from build123d import *

# Parameters (mm, degrees)
DODANIE_WYCI_GNI_CIE1_DEPTH = 45


with BuildPart() as part:
    # Szkic1 → Dodanie-wyciągnięcie1 (new body)
    with BuildSketch(Plane(origin=(0, 0, 0), x_dir=(1, 0, 0), z_dir=(0, 1, 0))):
        with BuildLine():
            Line((0, 3.9), (2.839339828, 3.9))
            Line((2.839339828, 3.9), (5.5, 6.560660172))
            Line((5.5, 6.560660172), (5.5, 8.2))
            Line((5.5, 8.2), (3.1, 8.2))
            Line((3.1, 8.2), (3.1, 10))
            Line((3.1, 10), (8.5, 10))
            ThreePointArc((8.5, 10), (9.560660172, 9.560660172), (10, 8.5))
            Line((10, 8.5), (10, 3.1))
            Line((10, 3.1), (8.2, 3.1))
            Line((8.2, 3.1), (8.2, 5.5))
            Line((8.2, 5.5), (6.560660172, 5.5))
            Line((6.560660172, 5.5), (3.9, 2.839339828))
            Line((3.9, 2.839339828), (3.9, 0))
            Line((3.9, 0), (3.9, -2.839339828))
            Line((3.9, -2.839339828), (6.560660172, -5.5))
            Line((6.560660172, -5.5), (8.2, -5.5))
            Line((8.2, -5.5), (8.2, -3.1))
            Line((8.2, -3.1), (10, -3.1))
            Line((10, -3.1), (10, -8.5))
            ThreePointArc((10, -8.5), (9.560660172, -9.560660172), (8.5, -10))
            Line((8.5, -10), (3.1, -10))
            Line((3.1, -10), (3.1, -8.2))
            Line((3.1, -8.2), (5.5, -8.2))
            Line((5.5, -8.2), (5.5, -6.560660172))
            Line((5.5, -6.560660172), (2.839339828, -3.9))
            Line((2.839339828, -3.9), (0, -3.9))
            Line((0, -3.9), (-2.839339828, -3.9))
            Line((-2.839339828, -3.9), (-5.5, -6.560660172))
            Line((-5.5, -6.560660172), (-5.5, -8.2))
            Line((-5.5, -8.2), (-3.1, -8.2))
            Line((-3.1, -8.2), (-3.1, -10))
            Line((-3.1, -10), (-8.5, -10))
            ThreePointArc((-8.5, -10), (-9.560660172, -9.560660172), (-10, -8.5))
            Line((-10, -8.5), (-10, -3.1))
            Line((-10, -3.1), (-8.2, -3.1))
            Line((-8.2, -3.1), (-8.2, -5.5))
            Line((-8.2, -5.5), (-6.560660172, -5.5))
            Line((-6.560660172, -5.5), (-3.9, -2.839339828))
            Line((-3.9, -2.839339828), (-3.9, 0))
            Line((-3.9, 0), (-3.9, 2.839339828))
            Line((-3.9, 2.839339828), (-6.560660172, 5.5))
            Line((-6.560660172, 5.5), (-8.2, 5.5))
            Line((-8.2, 5.5), (-8.2, 3.1))
            Line((-8.2, 3.1), (-10, 3.1))
            Line((-10, 3.1), (-10, 8.5))
            ThreePointArc((-10, 8.5), (-9.560660172, 9.560660172), (-8.5, 10))
            Line((-8.5, 10), (-3.1, 10))
            Line((-3.1, 10), (-3.1, 8.2))
            Line((-3.1, 8.2), (-5.5, 8.2))
            Line((-5.5, 8.2), (-5.5, 6.560660172))
            Line((-5.5, 6.560660172), (-2.839339828, 3.9))
            Line((-2.839339828, 3.9), (0, 3.9))
        make_face()
        with BuildLine():
            ThreePointArc((2.5, 0), (1.767766953, 1.767766953), (0, 2.5))
            ThreePointArc((0, 2.5), (-1.767766953, 1.767766953), (-2.5, 0))
            ThreePointArc((-2.5, 0), (-1.767766953, -1.767766953), (0, -2.5))
            ThreePointArc((0, -2.5), (1.767766953, -1.767766953), (2.5, 0))
        make_face(mode=Mode.SUBTRACT)
    extrude(amount=DODANIE_WYCI_GNI_CIE1_DEPTH)


solid = part.part
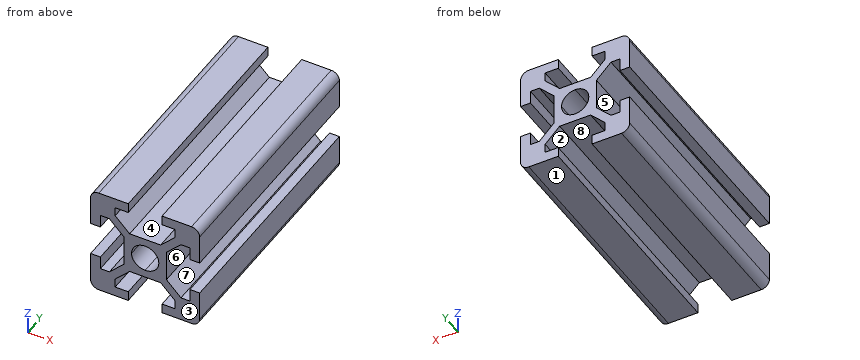
Design review of the part built by this model. Coordinates are the model's own, in mm. Face numbers are marked on the shaded views. A direction names the side the tool comes from. Coordinates: 2 decimals unless noted, no trailing zeros. Order: outer loops, then holes, each group sorted by start corner. A loop starts at its lowest first (then second) coordinate and runs counter-clockwise, first axis right, second up. Notation, with made-up numbers: (-17.75, 78.5) -> (-10.75, 78.5) arc R28 cw to (-10.75, 97.5) -> close; hole circle Ø4 at (70.25, -3). An arc over 180 degrees is marked (long way). Use one line per item in the form item = value. Start each with the question number.
(1) The part is to be moulded in two halves that separate along Z. For the marked faces 1, 2 and 3, say which applies: +Z half, -Z half, draft (parallel to the pull), parting line (faces both ways), or undercut.
(2) Insertion check: pin 1 (1.4 mm diameter, centred on y = 17, z = -9.5, fed in from +X); pin 2 (1 mm diameter, centred on x = -1.5, y = 8, fed in from -Z); pin 3 (3 mm diameter, centred on y = 27, z = 1, fed in from +X). Each pin has a flat end and moves straight along its axis. Give the tip position at first contact, or say it passes through.
(3) For probe 1 along Z at (x, y) = (-8, 14); probe 2 along Z at (x, y) = (-3.5, 35), list the stretches that pass through material, from the lowest coordinate up.
(4) Add section B-B on x = 7. State the section outline as (y, z) points, plus the area to 3 significant figures.
(5) Add section C-C on z = -5. State the section outline as (x, y) points.
(6) Add section A-A on z = -7.75. State the section outline as (x, y) points, plus the area to 3 significant figures.
(7) For the marked faces 4, 5, 6, 7 and 8, list the 3-axis set-ups (+Z, -Z, +X, -X, +Y, -Y) from which the entire face can be reached by the end or side of a thin tool; tool diameter is ignored.
Answer block:
q1.face_1 = -Z half
q1.face_2 = undercut
q1.face_3 = draft
q2.pin_1 = 9.97
q2.pin_2 = -3.9
q2.pin_3 = 3.9
q3.probe_1 = -10 to -5.5, 5.5 to 10
q3.probe_2 = -10 to -8.2, -4.56 to 4.56, 8.2 to 10
q4.outline = (0, -10) -> (45, -10) -> (45, -5.5) -> (0, -5.5) -> close; (0, 5.5) -> (45, 5.5) -> (45, 10) -> (0, 10) -> close
q4.area = 405 mm²
q5.outline = (-10, 0) -> (-8.2, 0) -> (-8.2, 45) -> (-10, 45) -> close; (-6.06, 0) -> (-3.94, 0) -> (-3.94, 45) -> (-6.06, 45) -> close; (3.94, 0) -> (6.06, 0) -> (6.06, 45) -> (3.94, 45) -> close; (8.2, 0) -> (10, 0) -> (10, 45) -> (8.2, 45) -> close
q6.outline = (-10, 0) -> (-5.5, 0) -> (-5.5, 45) -> (-10, 45) -> close; (5.5, 0) -> (10, 0) -> (10, 45) -> (5.5, 45) -> close
q6.area = 405 mm²
q7.face_4 = +Z, +Y, -Y
q7.face_5 = -X, +Y, -Y
q7.face_6 = +X, +Y, -Y
q7.face_7 = +Y, -Y
q7.face_8 = -Z, +Y, -Y
